from build123d import *

# Parameters (mm, degrees)
SKETCH2_W           = 23
SKETCH2_H           = 12.2
BOSS_EXTRUDE1_DEPTH = 5


with BuildPart() as part:
    # Sketch2 → Boss-Extrude1 (new body)
    with BuildSketch(Plane(origin=(0, 0, 0), x_dir=(1, 0, 0), z_dir=(0, 1, 0))):
        Polygon((-154.967912227, 159.789086559), (-80.967912227, 159.789086559), (-63.290242697, 177.466756088), (-50.420899279, 164.597412671), (-68.098568809, 146.919743141), (-68.098568809, 94.019743141), (-43.098568809, 94.019743141), (-43.098568809, 75.819743141), (-68.098568809, 75.819743141), (-68.098568809, 22.919743141), (-50.420899279, 5.242073612), (-63.290242697, -7.627269806), (-80.967912227, 10.050399724), (-154.967912227, 10.050399724), (-172.645581756, -7.627269806), (-185.514925174, 5.242073612), (-167.837255644, 22.919743141), (-167.837255644, 75.819743141), (-192.837255644, 75.819743141), (-192.837255644, 94.019743141), (-167.837255644, 94.019743141), (-167.837255644, 146.919743141), (-185.514925174, 164.597412671), (-172.645581756, 177.466756088), align=None)
        Polygon((-171.231368194, 171.809901839), (-154.967912227, 155.546445872), (-163.678194925, 146.836163173), (-179.941650892, 163.099619141), align=None, mode=Mode.SUBTRACT)
        with Locations((-176.337255644, 84.919743141)):
            Rectangle(SKETCH2_W, SKETCH2_H, mode=Mode.SUBTRACT)
        Polygon((-80.967912227, 155.546445872), (-72.257629528, 146.836163173), (-55.994173561, 163.099619141), (-64.704456259, 171.809901839), align=None, mode=Mode.SUBTRACT)
        Polygon((-64.704456259, -1.970415557), (-80.967912227, 14.293040411), (-72.257629528, 23.003323109), (-55.994173561, 6.739867142), align=None, mode=Mode.SUBTRACT)
        Polygon((-154.967912227, 14.293040411), (-163.678194925, 23.003323109), (-179.941650892, 6.739867142), (-171.231368194, -1.970415557), align=None, mode=Mode.SUBTRACT)
        with Locations((-59.598568809, 84.919743141)):
            Rectangle(SKETCH2_W, SKETCH2_H, mode=Mode.SUBTRACT)
    extrude(amount=BOSS_EXTRUDE1_DEPTH)


solid = part.part
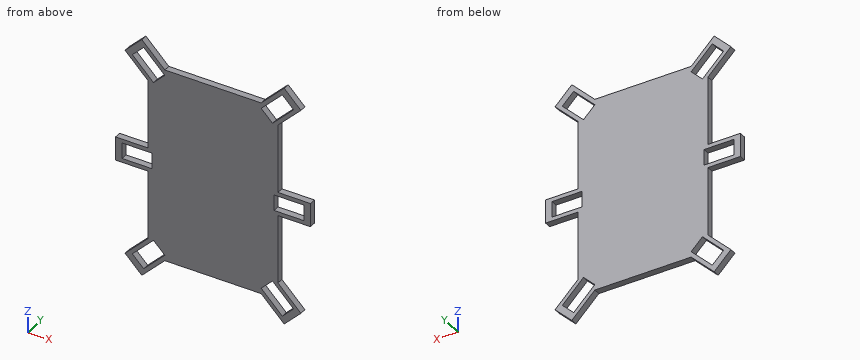
Geometry: final body of the model. Coordinates: model frame, mm. Give positions to 0.01 mm unless a question says otherwise; leave off trailing zeros. Order: outer loops, then holes, each group sorted by start corner. A loop starts at its lowest first (then second) coordinate and runs counter-clockwise, first axis right, second up. Notation, with made-up numbers: (-28, 2.25) -> (-21, 2.25) arc R30 cw to (-21, 24.25) -> close; hole circle Ø3 at (11, 21.25). An arc over 180 degrees is marked (long way). Answer as a JSON object with one key per item and string values.
Q1. Section D-D (z = -143). Output: boundary loops of the cut face in (x, y), plus the area to 3 significant figures.
Entries:
{"outline": "(-167.84, 0) -> (-68.1, 0) -> (-68.1, 5) -> (-167.84, 5) -> close", "area": "499 mm^2"}
Q2. First-contact query: pin 1 (1.5 mm diameter, centred on x = -160.5, z = -92.5, fed in from -Y); pin 2 (1 mm diameter, centred on y = 3, z = -127.5, fed in from -X); pin 3 (2.5 mm diameter, centred on x = -131.5, y = 3.5, fed in from +Z); pin 4 (1.5 mm diameter, centred on x = -183.5, y = 3, fed in from +Z). Flat tips, straight axial feed; report the tip coordinate or a pass-through.
Entries:
{"pin 1": "stops at y = 0", "pin 2": "stops at x = -167.84", "pin 3": "stops at z = -10.05", "pin 4": "stops at z = -2.48"}
Q3. Section C-C (y = 1.95). State how many separate pieces and enclosed holes the cut face has, plus the area to 3 significant figures.
Entries:
{"separate pieces": "1", "enclosed holes": "6", "area": "15,600 mm^2"}
Q4. Material intervals for probe 1 along Z at (x, y) = (-181, 1.95); probe 2 along Z at (x, y) = (-186, 0.6); probe 3 along Z at (x, y) = (-179, 3.8), sorted ascending.
Entries:
{"probe 1": "z = -169.11 to -160.08, -94.02 to -91.02, -78.82 to -75.82, -9.76 to -0.73", "probe 2": "z = -94.02 to -91.02, -78.82 to -75.82", "probe 3": "z = -171.11 to -164.04, -162.16 to -158.08, -94.02 to -91.02, -78.82 to -75.82, -11.76 to -7.68, -5.8 to 1.27"}
Q5. Section B-B (x = -59.5). Output: boundary loops of the cut face in (y, z).
Entries:
{"outline": "(0, -173.68) -> (5, -173.68) -> (5, -166.61) -> (0, -166.61) -> close; (0, -159.59) -> (5, -159.59) -> (5, -155.52) -> (0, -155.52) -> close; (0, -94.02) -> (5, -94.02) -> (5, -91.02) -> (0, -91.02) -> close; (0, -78.82) -> (5, -78.82) -> (5, -75.82) -> (0, -75.82) -> close; (0, -14.32) -> (5, -14.32) -> (5, -10.25) -> (0, -10.25) -> close; (0, -3.23) -> (5, -3.23) -> (5, 3.84) -> (0, 3.84) -> close"}
Q6. Section A-A (z = -21). Output: boundary loops of the cut face in (x, y).
Entries:
{"outline": "(-169.76, 0) -> (-165.68, 0) -> (-165.68, 5) -> (-169.76, 5) -> close; (-161.67, 0) -> (-74.26, 0) -> (-74.26, 5) -> (-161.67, 5) -> close; (-70.25, 0) -> (-66.18, 0) -> (-66.18, 5) -> (-70.25, 5) -> close"}
